```python
from build123d import *

# Parameters (mm, degrees)
F0_R     = 109.855
F1_DEPTH = 109.855
F3_D     = 194.31
F3_DEPTH = 50.8
F3_TIP   = 58.3766134416
F4_R     = 101.6


with BuildPart() as f1:
    # F0 (on Top) → F1 (new body)
    with BuildSketch(Plane.XY):
        Circle(F0_R)
    extrude(amount=F1_DEPTH)

    # F3
    with Locations(Plane.XY.offset(109.855)):
        with Locations((0, 0)):
            Hole(F3_D / 2, depth=F3_DEPTH)
            with Locations((0, 0, -(F3_DEPTH + F3_TIP / 2))):  # 118° drill point
                Cone(0, F3_D / 2, F3_TIP, mode=Mode.SUBTRACT)

    # F4
    f4_edges = [f1.edges().sort_by_distance(p)[0] for p in [
        (-109.855, 0, 0),
    ]]
    fillet(f4_edges, radius=F4_R)


solid = f1.part
```
Design review of the part built by this model. Coordinates are the model's own, in mm. Coordinates: 2 decimals unless noted, no trailing zeros. Answer in a Markdown table with one row per item.
(1) The part is to be moulded in two halves that separate along Y. For faces 1 (the flat face through (0, 0, 0)), 2 (the cylindrical face through (21.061, -94.845, 84.099)), 3 (the conical face through (16.093, 5.068, 10.816)), 4 (the cylindrical face through (-14.3, 108.92, 105.67)), say which applies: released by +Y, released by -Y, zero draft, split by the parting line, or undercut.
Checked values:
| item | result |
|---|---|
| face 1 | zero draft |
| face 2 | undercut |
| face 3 | undercut |
| face 4 | split by the parting line |
(2) Clearance check with flat-ended pins moving along their axes: pin 1 (12 mm diameter, centred on y = 83, z = 51.5, fed in from -X); pin 2 (12 mm diameter, centred on x = 68, z = 89.5, fed in from -Y); pin 3 (1.5 mm diameter, centred on x = 36, z = 91, fed in from +Y). State where each tip first meets the part, or that it passes through.
Checked values:
| item | result |
|---|---|
| pin 1 | x = -60.06 |
| pin 2 | y = -89.89 |
| pin 3 | y = 103.47 |
(3) Wall thickness on line 1 along X through (y, z) = (0, 100) (3 decimals); line 2 along X through (y, z) = (52, 93); line 3 along Y through (x, z) = (21, 71.5): over which ranges is each line inside the solid? List them lowest first. Write a range as from..to.
Checked values:
| item | result |
|---|---|
| line 1 | -109.842..-97.155, 97.155..109.842 |
| line 2 | -96.35..-82.07, 82.07..96.35 |
| line 3 | -103.18..-94.86, 94.86..103.18 |
